Could you check a few things on this drawing? It's one solid part, dimensions in mm from its lowest x, y, z. A direction names the side the tool comes from. Give positions to 0.01 mm unless a question says otherwise; leave off trailing zeros. Write each loop counter-clockwise with the first axis right and the second up, starting at its lowest first coordinate (ties: lowest second). Pieces come first, ordered by that corner, then holes.
1. Suppose I cut it at C-C (z = 9). Please give me the cut outline in (x, y) (1 decimal).
2. Suppose I cut it at A-A (z = 26). Please give me the cut outline in (x, y) (1 decimal).
3. If I drill on probe 1 along Z at (x, y) = (17, 2.5) (1 decimal); probe 2 along X at (y, z) = (1.15, 25.5) (1 decimal); probe 3 along X at (y, z) = (1.4, 18.5) (1 decimal), over which ranges is the centre line in solid material (lowest first)?
4. On a 3-axis mill with a long thin cutter (end or side, diameter ignored), from which of +Z, -Z, +X, -X, +Y, -Y can I reach the whole of each face in a straight line? I mean the marked faces 5 and 6. Say none if no direction works.
5. I'm going to push flat-ended pins straight in: pin 1 (1.6 mm diameter, centred on x = 21.5, y = 1.5, fed in from -Z); pin 2 (1.6 mm diameter, centred on y = 1, z = 10.5, fed in from -X) (1 decimal); pin 3 (0.5 mm diameter, centred on y = 2, z = 21.5, fed in from -X). Where does each tip first touch, or does it pass through?
6. Suppose I cut it at B-B (y = 0.55). Please give me the cut outline in (x, z) (1 decimal), and give its area (3 significant figures).
7. Suppose I cut it at D-D (x = 23.5). Please give me the cut outline in (y, z) (1 decimal).
8. Thinking about a two-plate mould opening in Z: for the marked faces 1, 2, 3 and 4, which applies, pulls with the +Z half, pulls with the -Z half, needs draft (parallel to the pull), parting line crosses it, or undercut?
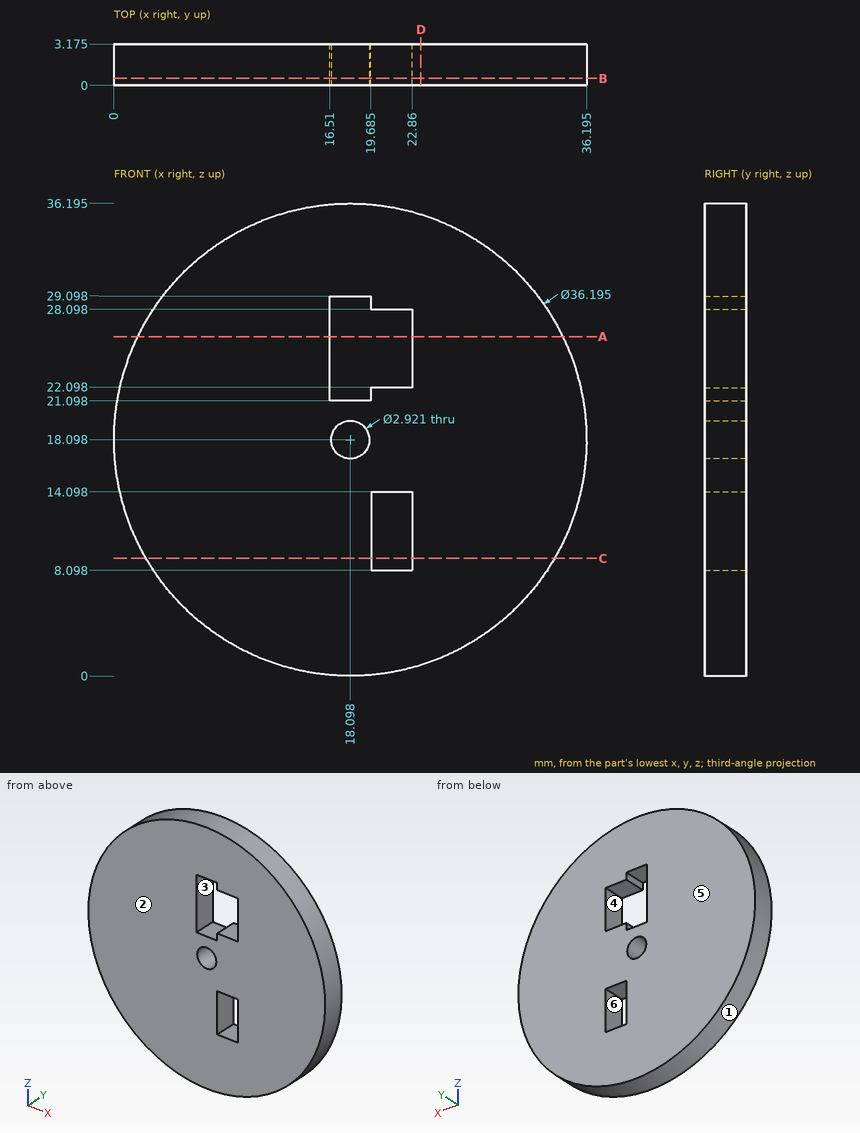
Checks:
1. outline: (2.5, 0) - (19.7, 0) - (19.7, 3.2) - (2.5, 3.2) - close; (22.9, 0) - (33.7, 0) - (33.7, 3.2) - (22.9, 3.2) - close
2. outline: (1.8, 0) - (16.5, 0) - (16.5, 3.2) - (1.8, 3.2) - close; (22.9, 0) - (34.4, 0) - (34.4, 3.2) - (22.9, 3.2) - close
3. probe 1: z = 0 to 17.1, 19.1 to 21.1, 29.1 to 36.2
3. probe 2: x = 1.6 to 16.5, 22.9 to 34.6
3. probe 3: x = 0 to 16.7, 19.5 to 36.2
4. face 5: +Z, -Z, +X, -X, +Y
4. face 6: +Y, -Y
5. pin 1: stops at z = 0.19
5. pin 2: stops at x = 1.3
5. pin 3: stops at x = 0.28
6. outline: circle Ø36.2 at (18.1, 18.1); hole (16.5, 21.1) - (19.7, 21.1) - (19.7, 22.1) - (22.9, 22.1) - (22.9, 28.1) - (19.7, 28.1) - (19.7, 29.1) - (16.5, 29.1) - close; hole circle Ø2.9 at (18.1, 18.1); hole (19.7, 8.1) - (22.9, 8.1) - (22.9, 14.1) - (19.7, 14.1) - close
6. area: 959 mm2
7. outline: (0, 0.8) - (3.2, 0.8) - (3.2, 35.4) - (0, 35.4) - close
8. face 1: parting line crosses it
8. face 2: needs draft
8. face 3: undercut
8. face 4: undercut
